from build123d import *

# Parameters (mm, degrees)
F1_DEPTH      = 60
F2_T1_DEPTH   = 128.3050587773
F2_T3_DEPTH   = 87.2325127198
F2_T5_DEPTH   = 83.2679866238
F3_W          = 31.2075465918
F3_H          = 53.4305032343
F4_DEPTH      = 47.1568533609
F4_DEPTH_BACK = 100


# Not quite as in the source:
# - a fillet or chamfer that OpenCascade refuses, or shapes differently, is made with other operations: its cross-section is extruded or revolved along the edge and cut away or added


with BuildPart() as f1:
    # F0 (on Front) → F1 (new body)
    with BuildSketch(Plane.XZ):
        Polygon((-43.1315037153, 54.6031631236), (-47.1558533609, 53.3990226686), (-38.1231829524, 0), (15.0101743639, 0), (17.1355064958, -2.9223344754), (-27.4965111166, -40.6470149755), (-38.7919515192, -50.1943512397), (51.1408522725, -50.1943512397), (51.1408522725, -47.0230206847), (-30.1531795412, -47.0230206847), (19.4947316054, -5.0587160063), (29.0376522148, 3.0073238074), (-34.4038493931, 3.0073238074), align=None)
    extrude(amount=F1_DEPTH)

    # F2: fillet of radius 5 on 3 edges, made by hand

    # F2_s2 → F2_t1 (cut)
    with BuildSketch(Plane.XZ.offset(-34.1525293886)):
        with BuildLine():
            ThreePointArc((18.6043132835, -5.8113314716), (20.0720252356, -0.274141409), (15.3766404593, 3.0073238074))
            Line((15.3766404593, 3.0073238074), (29.0376522148, 3.0073238074))
            Line((29.0376522148, 3.0073238074), (18.6043132835, -5.8113314716))
        make_face()
    extrude(amount=F2_T1_DEPTH, mode=Mode.SUBTRACT)

    # F2_s4 → F2_t3 (cut)
    with BuildSketch(Plane.XZ.offset(-13.6162563599)):
        with BuildLine():
            ThreePointArc((-47.1558533609, 53.3990226686), (-43.9268794892, 52.21892637), (-42.2231091456, 49.2329481124))
            Line((-42.2231091456, 49.2329481124), (-43.1315037153, 54.6031631236))
            Line((-43.1315037153, 54.6031631236), (-47.1558533609, 53.3990226686))
        make_face()
    extrude(amount=F2_T3_DEPTH, mode=Mode.SUBTRACT)

    # F2_s6 → F2_t5 (cut)
    with BuildSketch(Plane.XZ.offset(-11.6339933119)):
        with BuildLine():
            ThreePointArc((51.1408522725, -50.1943512397), (49.3029833415, -47.8912324989), (46.4872549478, -47.0230206847))
            Line((46.4872549478, -47.0230206847), (51.1408522725, -47.0230206847))
            Line((51.1408522725, -47.0230206847), (51.1408522725, -50.1943512397))
        make_face()
    extrude(amount=F2_T5_DEPTH, mode=Mode.SUBTRACT)

    # F3 (on Right) → F4 (cut, two sides)
    with BuildSketch(Plane.YZ) as f4_sk:
        with Locations((-29.6471677721, -47.0001557842)):
            Rectangle(F3_W, F3_H)
    extrude(amount=-F4_DEPTH, mode=Mode.SUBTRACT)
    extrude(f4_sk.sketch, amount=F4_DEPTH_BACK, mode=Mode.SUBTRACT)


solid = f1.part
CAD build for the part. Positions are in the model's coordinates, mm. A direction names the side the tool comes from. Round coordinates to 2 decimals unless told otherwise and drop trailing zeros. Loops run counter-clockwise (first coordinate to the right, second up) from the corner with the lowest first, then second, coordinate; pieces in that order, holes last. Notation, with made-up numbers: (49.5, 2) - (97.5, 2) arc R20 cw to (97.5, 18) - close; hole circle Ø5 at (55.25, 89). An arc over 180 degrees is marked (long way). Put each result on its own line as item: value.
1. 3-axis set-ups, long thin cutter, end or side, ignore diameter. For faces 4 (the flat face through (-12, -30, 0)), 5 (the flat face through (-9, -30, 3.007)), 6 (the flat face through (9, -53, -47.023)), 7 (the flat face through (-1, -30, -20.285)): which of +Z, -Z, +X, -X, +Y, -Y reach the whole face in a straight line?
Geometry check:
face 4: -X, +Y, -Y
face 5: +Z, +X, +Y, -Y
face 6: +X, +Y, -Y
face 7: -Z, +X, -X
2. Pin check, flat tips, straight feed: P1, Ø12, axis at x = -0.5, y = -53, coming from the +Z side; P2, Ø2.5, axis at x = -1.5, y = -25, coming from the -Z side; P3, Ø1.5, axis at x = -36, y = -35, coming from the -Z side; P4, Ø8, axis at x = 33.5, y = -38, coming from the -Z side. Stop position of each tip, or through.
Geometry check:
P1: z = 3.01
P2: z = -20.28
P3: z = 0
P4: through
3. Two-plate mould, pull along Y, no slides. Class faces 1 (the flat face through (-2, -60, -21)), 2 (the flat face through (-42.703, -29.58, 27.073)), 3 (the flat face through (-0.3, -45.251, -47.5)): released by +Y, released by -Y, zero draft, split by the parting line, or undercut.
Geometry check:
face 1: released by -Y
face 2: zero draft
face 3: undercut
4. Slice it at D-D on x = 12. List the corners of the cut face in (y, z).
Geometry check:
outline: (-60, -50.19) - (-45.25, -50.19) - (-45.25, -47.02) - (-60, -47.02) - close; (-60, -11.39) - (0, -11.39) - (0, -7.26) - (-60, -7.26) - close; (-60, 0) - (0, 0) - (0, 3.01) - (-60, 3.01) - close; (-14.04, -50.19) - (0, -50.19) - (0, -47.02) - (-14.04, -47.02) - close
5. Wall check: line 1 (Z direction, x = -29, y = -54); line 2 (Z direction, x = -18, y = -47); line 3 (Z direction, x = 9, y = -34). Give the ranges that are in metal, low to high.
Geometry check:
line 1: -50.19 to -47.02, -46.05 to -41.92, 0 to 3.01
line 2: -50.19 to -47.02, -36.75 to -32.62, 0 to 3.01
line 3: -13.93 to -9.8, 0 to 3.01
6. Slice it at B-B on y = -19.5. List the corners of the cut face in (x, z), and give its area (3 significant figures).
Geometry check:
outline: (-47.16, 53.4) - (-38.12, 0) - (15.01, 0) - (17.14, -2.92) - (-3.41, -20.28) - (1.48, -20.28) - (18.6, -5.81) arc R5 ccw to (15.38, 3.01) - (-34.4, 3.01) - (-42.22, 49.23) arc R5 ccw to start
area: 476 mm²
7. Slice it at A-A on x = 39.5. List the corners of the cut face in (y, z), and give its area (3 significant figures).
Geometry check:
outline: (-60, -50.19) - (-45.25, -50.19) - (-45.25, -47.02) - (-60, -47.02) - close; (-14.04, -50.19) - (0, -50.19) - (0, -47.02) - (-14.04, -47.02) - close
area: 91.3 mm²
8. Slice it at C-C on x = -25.5. List the corners of the cut face in (y, z), and give its area (3 significant figures).
Geometry check:
outline: (-60, -50.19) - (-45.25, -50.19) - (-45.25, -47.02) - (-60, -47.02) - close; (-60, -43.09) - (-45.25, -43.09) - (-45.25, -38.96) - (-60, -38.96) - close; (-60, 0) - (0, 0) - (0, 3.01) - (-60, 3.01) - close; (-14.04, -50.19) - (0, -50.19) - (0, -47.02) - (-14.04, -47.02) - close; (-14.04, -43.09) - (0, -43.09) - (0, -38.96) - (-14.04, -38.96) - close
area: 391 mm²
